Source: three-view drawing plus pictorial views. Frame: mm from the lowest corner of the part. Coordinates: 2 decimals unless noted, no trailing zeros. Loops run counter-clockwise (first coordinate to the right, second up) from the corner with the lowest first, then second, coordinate; pieces in that order, holes last. Notation, with made-up numbers: M 51.25,49 L 79.25,49 A14 cw 79.25,70 Z; hole C 13.5,-21.75 d11. An arc over 180 degrees is marked long. Use a Markdown table: item, result. Add a question column.
1. Section D-D on y = 82.5. Output: boundary loops of the cut face in (x, z).
2. Section A-A on y = 111. Output: boundary loops of the cut face in (x, z) (1 decimal).
3. Section B-B on z = 1.4. Output: boundary loops of the cut face in (x, y) (1 decimal), then the cut area to 3 significant figures.
4. Line query: L1, parallel to X at y = 66.5, z = 2.1 (1 decimal); L2, parallel to Y at x = 136, z = 1.85 (1 decimal); L3, parallel to Y at x = 107.5, z = 1.4. Output: solid intervals per line, ascending. Write a range as [from, to].
5. Section C-C on x = 28.5. Output: boundary loops of the cut face in (y, z) (1 decimal).
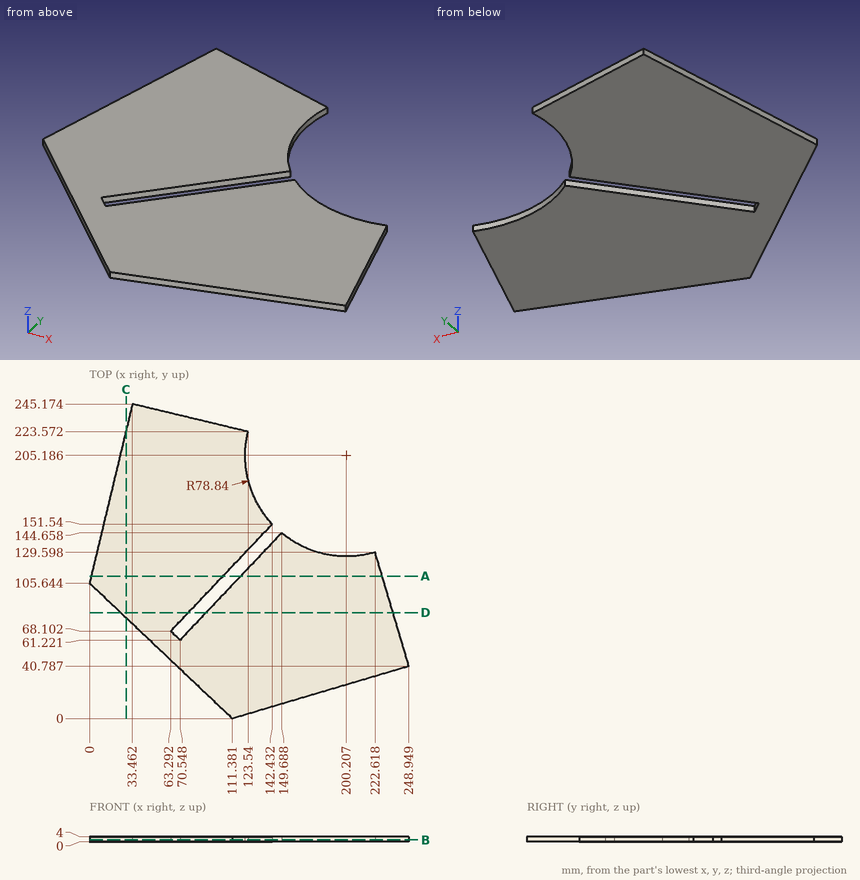
Answers below:
| question | item | result |
|---|---|---|
| 1 | outline | M 24.4,0 L 76.95,0 L 76.95,4 L 24.4,4 Z; M 90.73,0 L 236.58,0 L 236.58,4 L 90.73,4 Z |
| 2 | outline | M 1.3,0 L 104,0 L 104,4 L 1.3,4 Z; M 117.8,0 L 228.1,0 L 228.1,4 L 117.8,4 Z |
| 3 | outline | M 0,105.6 L 111.4,0 L 248.9,40.8 L 222.6,129.6 A78.8 cw 149.7,144.7 L 70.5,61.2 L 63.3,68.1 L 142.4,151.5 A78.8 cw 123.5,223.6 L 33.5,245.2 Z |
| 3 | area | 33,100 mm² |
| 4 | L1 | x = [41.3, 65], [75.6, 241.3] |
| 4 | L2 | y = [7.3, 130.2], [144.8, 159.4] |
| 4 | L3 | y = [3.68, 100.18], [114.71, 227.42] |
| 5 | outline | M 78.6,0 L 224.5,0 L 224.5,4 L 78.6,4 Z |
